from build123d import *

# Parameters (mm, degrees)
SKETCH1_W           = 50
SKETCH1_H           = 40
BOSS_EXTRUDE1_DEPTH = 3
FILLET1_R           = 4
SKETCH2_R           = 1.5
CUT_EXTRUDE1_DEPTH  = 3
SKETCH3_R           = 1.5
CUT_EXTRUDE3_DEPTH  = 3


with BuildPart() as part:
    # Sketch1 → Boss-Extrude1 (new body)
    with BuildSketch(Plane(origin=(0, 0, 0), x_dir=(1, 0, 0), z_dir=(0, 1, 0))):
        Rectangle(SKETCH1_W, SKETCH1_H)
    extrude(amount=BOSS_EXTRUDE1_DEPTH)

    # Fillet1
    fillet1_edges = [part.edges().sort_by_distance(p)[0] for p in [
        (25, 1.5, 20),
        (-25, 1.5, 20),
        (-25, 1.5, -20),
        (25, 1.5, -20),
    ]]
    fillet(fillet1_edges, radius=FILLET1_R)

    # Sketch2 → Cut-Extrude1 (cut)
    with BuildSketch(Plane(origin=(0, 0, 0), x_dir=(1, 0, 0), z_dir=(0, 1, 0))):
        with Locations(Location((-20, 0, 0), (0, 0, 270))):
            Circle(SKETCH2_R)
        with Locations(Location((20, 0, 0), (0, 0, 270))):
            Circle(SKETCH2_R)
    extrude(amount=CUT_EXTRUDE1_DEPTH, mode=Mode.SUBTRACT)

    # Sketch3 → Cut-Extrude3 (cut)
    with BuildSketch(Plane(origin=(0, 0, 0), x_dir=(1, 0, 0), z_dir=(0, 1, 0))):
        with Locations(Location((-20, -15, 0), (0, 0, 270))):
            Circle(SKETCH3_R)
        with Locations(Location((20, -15, 0), (0, 0, 270))):
            Circle(SKETCH3_R)
        with Locations(Location((20, 15, 0), (0, 0, 270))):
            Circle(SKETCH3_R)
        with Locations(Location((-20, 15, 0), (0, 0, 270))):
            Circle(SKETCH3_R)
    extrude(amount=CUT_EXTRUDE3_DEPTH, mode=Mode.SUBTRACT)


solid = part.part
Part model, mm, in its own coordinate system. Coordinates: 2 decimals unless noted, no trailing zeros. Write each loop counter-clockwise with the first axis right and the second up, starting at its lowest first coordinate (ties: lowest second). Pieces come first, ordered by that corner, then holes. Notation, with made-up numbers: M -17.75,-19.75 L 30.25,-19.75 A20 cw 30.25,-7.75 Z; hole C 11.5,26.25 d2. An arc over 180 degrees is marked long. Return JSON: item names as keys, results as strings.
1. Saw through at A-A, the plane x = -20. Write the cut outline in (y, z), then the cut area to 3 significant figures.
Determined:
{"outline": "M 0,-20 L 3,-20 L 3,-16.5 L 0,-16.5 Z; M 0,-13.5 L 3,-13.5 L 3,-1.5 L 0,-1.5 Z; M 0,1.5 L 3,1.5 L 3,13.5 L 0,13.5 Z; M 0,16.5 L 3,16.5 L 3,20 L 0,20 Z", "area": "93.0 mm²"}
2. Flat gauge pin, fed straight in: pin 1 Ø3.5 at (x, z) = (-20, 15) entering from -Y. Where does the tip first touch, or does it go through?
Determined:
{"pin 1": "y = 0"}
3. Saw through at C-C, the plane y = 0.6. Write the cut outline in (x, z).
Determined:
{"outline": "M -25,-16 A4 ccw -21,-20 L 21,-20 A4 ccw 25,-16 L 25,16 A4 ccw 21,20 L -21,20 A4 ccw -25,16 Z; hole C -20,-15 d3; hole C -20,0 d3; hole C -20,15 d3; hole C 20,-15 d3; hole C 20,0 d3; hole C 20,15 d3"}
4. Saw through at B-B, the plane z = 15. Write the cut outline in (x, y).
Determined:
{"outline": "M -25,0 L -21.5,0 L -21.5,3 L -25,3 Z; M -18.5,0 L 18.5,0 L 18.5,3 L -18.5,3 Z; M 21.5,0 L 25,0 L 25,3 L 21.5,3 Z"}
5. Probe L1, parallel to X at y = 1.2, z = 15; L2, parallel to X at y = 1.6, z = -16. List the from-to ranges inside material, lowest first.
Determined:
{"L1": "-25 to -21.5, -18.5 to 18.5, 21.5 to 25", "L2": "-25 to -21.12, -18.88 to 18.88, 21.12 to 25"}
6. Pull direction X, two halves, no side cores. Call faces 1 (the face through (25, 1, 0)), 2 (the face through (21.265, 1.479, 0.806)), 3 (the face through (-23.859, 1.521, 18.797)), 4 (the face through (0, 0, 0)): pulls with the +X half, pulls with the -X half, needs draft (parallel to the pull), parting line crosses it, or undercut.
Determined:
{"face 1": "pulls with the +X half", "face 2": "undercut", "face 3": "pulls with the -X half", "face 4": "needs draft"}
